The model under review builds one solid part; all positions refer to its coordinate system, in mm. Face numbers are marked on the shaded views. A direction names the side the tool comes from. Round coordinates to 2 decimals unless told otherwise and drop trailing zeros. Write each loop counter-clockwise with the first axis right and the second up, starting at its lowest first coordinate (ties: lowest second). Pieces come first, ordered by that corner, then holes. Notation, with made-up numbers: (77.25, -26.5) - (112.25, -26.5) arc R19 ccw to (112.25, -10.5) - close; hole circle Ø1 at (88.5, 85.25). An arc over 180 degrees is marked (long way). One line per question, with ' | ' between items. Start each with the question number.
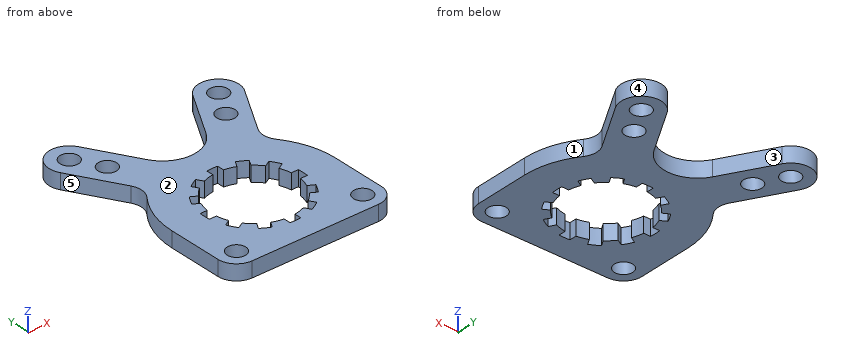
```python
from build123d import *

# Parameters (mm, degrees)
SALIENTE_EXTRUIR1_DEPTH = 10
CROQUIS2_R              = 6
CORTAR_EXTRUIR3_DEPTH   = 116.291439701


with BuildPart() as part:
    # Croquis1 → Saliente-Extruir1 (new body)
    with BuildSketch(Plane.XY):
        with BuildLine():
            Line((-59.758330249, 77.504464167), (-41.258330249, 45.461524227))
            ThreePointArc((-41.258330249, 45.461524227), (-39.675513612, 38.689212456), (-42.115133231, 32.176319754))
            ThreePointArc((-42.115133231, 32.176319754), (-50.205089688, 16.983785484), (-53, 0))
            Line((-53, 0), (-53, -35))
            ThreePointArc((-53, -35), (-49.485281374, -43.485281374), (-41, -47))
            Line((-41, -47), (41, -47))
            ThreePointArc((41, -47), (49.485281374, -43.485281374), (53, -35))
            Line((53, -35), (53, 0))
            ThreePointArc((53, 0), (50.205089688, 16.983785484), (42.115133231, 32.176319754))
            ThreePointArc((42.115133231, 32.176319754), (39.675513612, 38.689212456), (41.258330249, 45.461524227))
            Line((41.258330249, 45.461524227), (59.758330249, 77.504464167))
            ThreePointArc((59.758330249, 77.504464167), (55, 95.262794416), (37.241669751, 90.504464167))
            Line((37.241669751, 90.504464167), (19.052558883, 59))
            ThreePointArc((19.052558883, 59), (0, 48), (-19.052558883, 59))
            Line((-19.052558883, 59), (-37.241669751, 90.504464167))
            ThreePointArc((-37.241669751, 90.504464167), (-55, 95.262794416), (-59.758330249, 77.504464167))
        make_face()
    extrude(amount=SALIENTE_EXTRUIR1_DEPTH)

    # Croquis2 → Cortar-Extruir3 (cut, through all)
    with BuildSketch(Plane.XY.offset(10)):
        with Locations((-41, -35)):
            Circle(CROQUIS2_R)
        with Locations((41, -35)):
            Circle(CROQUIS2_R)
        with Locations((-48.5, 84.004464167)):
            Circle(CROQUIS2_R)
        with Locations((48.5, 84.004464167)):
            Circle(CROQUIS2_R)
        with Locations((-38.5, 66.683956091)):
            Circle(CROQUIS2_R)
        with Locations((38.5, 66.683956091)):
            Circle(CROQUIS2_R)
        with BuildLine():
            Line((-3.5, 31.808017857), (-3.5, 27.276363394))
            ThreePointArc((-3.5, 27.276363394), (-7.11752374, 26.562960223), (-10.607092784, 25.372023622))
            Line((-10.607092784, 25.372023622), (-12.872920015, 29.296551508))
            ThreePointArc((-12.872920015, 29.296551508), (-16, 27.712812921), (-18.935097842, 25.796551508))
            Line((-18.935097842, 25.796551508), (-16.66927061, 21.872023622))
            ThreePointArc((-16.66927061, 21.872023622), (-19.445436483, 19.445436483), (-21.872023622, 16.66927061))
            Line((-21.872023622, 16.66927061), (-25.796551508, 18.935097842))
            ThreePointArc((-25.796551508, 18.935097842), (-27.712812921, 16), (-29.296551508, 12.872920015))
            Line((-29.296551508, 12.872920015), (-25.372023622, 10.607092784))
            ThreePointArc((-25.372023622, 10.607092784), (-26.562960223, 7.11752374), (-27.276363394, 3.5))
            Line((-27.276363394, 3.5), (-31.808017857, 3.5))
            ThreePointArc((-31.808017857, 3.5), (-32, 0), (-31.808017857, -3.5))
            Line((-31.808017857, -3.5), (-27.276363394, -3.5))
            ThreePointArc((-27.276363394, -3.5), (-26.562960223, -7.11752374), (-25.372023622, -10.607092784))
            Line((-25.372023622, -10.607092784), (-29.296551508, -12.872920015))
            ThreePointArc((-29.296551508, -12.872920015), (-27.712812921, -16), (-25.796551508, -18.935097842))
            Line((-25.796551508, -18.935097842), (-21.872023622, -16.66927061))
            ThreePointArc((-21.872023622, -16.66927061), (-19.445436483, -19.445436483), (-16.66927061, -21.872023622))
            Line((-16.66927061, -21.872023622), (-18.935097842, -25.796551508))
            ThreePointArc((-18.935097842, -25.796551508), (-16, -27.712812921), (-12.872920015, -29.296551508))
            Line((-12.872920015, -29.296551508), (-10.607092784, -25.372023622))
            ThreePointArc((-10.607092784, -25.372023622), (-7.11752374, -26.562960223), (-3.5, -27.276363394))
            Line((-3.5, -27.276363394), (-3.5, -31.808017857))
            ThreePointArc((-3.5, -31.808017857), (0, -32), (3.5, -31.808017857))
            Line((3.5, -31.808017857), (3.5, -27.276363394))
            ThreePointArc((3.5, -27.276363394), (7.11752374, -26.562960223), (10.607092784, -25.372023622))
            Line((10.607092784, -25.372023622), (12.872920015, -29.296551508))
            ThreePointArc((12.872920015, -29.296551508), (16, -27.712812921), (18.935097842, -25.796551508))
            Line((18.935097842, -25.796551508), (16.66927061, -21.872023622))
            ThreePointArc((16.66927061, -21.872023622), (19.445436483, -19.445436483), (21.872023622, -16.66927061))
            Line((21.872023622, -16.66927061), (25.796551508, -18.935097842))
            ThreePointArc((25.796551508, -18.935097842), (27.712812921, -16), (29.296551508, -12.872920015))
            Line((29.296551508, -12.872920015), (25.372023622, -10.607092784))
            ThreePointArc((25.372023622, -10.607092784), (26.562960223, -7.11752374), (27.276363394, -3.5))
            Line((27.276363394, -3.5), (31.808017857, -3.5))
            ThreePointArc((31.808017857, -3.5), (32, 0), (31.808017857, 3.5))
            Line((31.808017857, 3.5), (27.276363394, 3.5))
            ThreePointArc((27.276363394, 3.5), (26.562960223, 7.11752374), (25.372023622, 10.607092784))
            Line((25.372023622, 10.607092784), (29.296551508, 12.872920015))
            ThreePointArc((29.296551508, 12.872920015), (27.712812921, 16), (25.796551508, 18.935097842))
            Line((25.796551508, 18.935097842), (21.872023622, 16.66927061))
            ThreePointArc((21.872023622, 16.66927061), (19.445436483, 19.445436483), (16.66927061, 21.872023622))
            Line((16.66927061, 21.872023622), (18.935097842, 25.796551508))
            ThreePointArc((18.935097842, 25.796551508), (16, 27.712812921), (12.872920015, 29.296551508))
            Line((12.872920015, 29.296551508), (10.607092784, 25.372023622))
            ThreePointArc((10.607092784, 25.372023622), (7.11752374, 26.562960223), (3.5, 27.276363394))
            Line((3.5, 27.276363394), (3.5, 31.808017857))
            ThreePointArc((3.5, 31.808017857), (0, 32), (-3.5, 31.808017857))
        make_face()
    extrude(amount=-CORTAR_EXTRUIR3_DEPTH, mode=Mode.SUBTRACT)


solid = part.part
```
1. Add section B-B, the plane x = 9. Write out the cut boundary in (y, z).
2. The part is to be moulded in two halves that separate along Y. For the marked faces 1, 2 and 3, say which applies: pulls with the +Y half, pulls with the -Y half, needs draft (parallel to the pull), parting line crosses it, or undercut.
3. Add section D-D, the plane y = 43. Write out the cut boundary in (x, z).
4. Machinability: for the marked faces 4 and 5, which of the approach directions +Z, -Z, +X, -X, +Y, -Y give a long, thin tool a straight path to every point of the face, cutting with its end or side? Answer none if there is none.
5. Wall thickness on line 1 along X through (y, z) = (83, 7.75); line 2 along X through (y, z) = (89.5, 4.25); line 3 along Y through (x, z) = (-29, 5.5): over which ranges is each line inside the solid? List them lowest first. Write a range as [from, to].
6. Add section A-A, the plane y = 65. Write out the cut boundary in (x, z).
7. Clearance check with flat-ended pins moving along their axes: P1, Ø2.5, axis at y = -29.5, z = 6.5, coming from the -X side; P2, Ø3, axis at x = 1, z = 8.5, coming from the +Y side; P3, Ø14, axis at x = -38.5, y = 66.68, coming from the -Z side; P4, Ø9.5, axis at x = 38.5, y = 66.68, coming from the +Z side. State where each tip first meets the part, or that it passes through.
8. Add section C-C, the plane z = 4.25. State how many separate pieces and enclosed holes the cut face has, then the cut area to 3 significant figures.
Geometry check:
1) outline: (-47, 0) - (-25.99, 0) - (-25.99, 10) - (-47, 10) - close; (25.99, 0) - (49.93, 0) - (49.93, 10) - (25.99, 10) - close
2) face 1: undercut | face 2: needs draft | face 3: pulls with the +Y half
3) outline: (-40.18, 0) - (40.18, 0) - (40.18, 10) - (-40.18, 10) - close
4) face 4: +Z, -Z | face 5: +Z, -Z, -X
5) line 1: x = [-61.46, -54.42], [-42.58, -32.91], [32.91, 42.58], [54.42, 61.46] | line 2: x = [-60.28, -50.91], [-46.09, -36.66], [36.66, 46.09], [50.91, 60.28] | line 3: y = [-47, -13.53], [-12.7, -3.5], [3.5, 12.7], [13.53, 76.23]
6) outline: (-52.54, 0) - (-44.26, 0) - (-44.26, 10) - (-52.54, 10) - close; (-32.74, 0) - (-22.52, 0) - (-22.52, 10) - (-32.74, 10) - close; (22.52, 0) - (32.74, 0) - (32.74, 10) - (22.52, 10) - close; (44.26, 0) - (52.54, 0) - (52.54, 10) - (44.26, 10) - close
7) P1: stops at x = -53 | P2: stops at y = 48.14 | P3: stops at z = 0 | P4: passes through
8) separate pieces: 1 | enclosed holes: 7 | area: 8,700 mm2
